from build123d import *

# Parameters (mm, degrees)
SKETCH1_R           = 29.25
SKETCH1_R_2         = 22.025
BOSS_EXTRUDE1_DEPTH = 7
CUT_EXTRUDE1_START  = 7
SKETCH1_3_R         = 1.55
CUT_EXTRUDE1_DEPTH  = 4
SKETCH4_R           = 22.25
SKETCH4_R_2         = 21
BOSS_EXTRUDE2_DEPTH = 1
SKETCH3_R           = 1.55
CUT_EXTRUDE2_DEPTH  = 42.953843686
CHAMFER1_SIZE       = 0.5


with BuildPart() as part:
    # Sketch1 → Boss-Extrude1 (new body)
    with BuildSketch(Plane.XY):
        Circle(SKETCH1_R)
        Circle(SKETCH1_R_2, mode=Mode.SUBTRACT)
    extrude(amount=BOSS_EXTRUDE1_DEPTH)

    # Sketch1<3> → Cut-Extrude1 (cut)
    with BuildSketch(Plane.XY.offset(CUT_EXTRUDE1_START)):
        with Locations((0, 25)):
            Circle(SKETCH1_3_R)
        with Locations((10.847093478, 22.524221698)):
            Circle(SKETCH1_3_R)
        with Locations((19.545787062, 15.587245046)):
            Circle(SKETCH1_3_R)
        with Locations((24.373197805, 5.563023349)):
            Circle(SKETCH1_3_R)
        with Locations((24.373197805, -5.563023349)):
            Circle(SKETCH1_3_R)
        with Locations((19.545787062, -15.587245046)):
            Circle(SKETCH1_3_R)
        with Locations((10.847093478, -22.524221698)):
            Circle(SKETCH1_3_R)
        with Locations((0, -25)):
            Circle(SKETCH1_3_R)
        with Locations((-10.847093478, -22.524221698)):
            Circle(SKETCH1_3_R)
        with Locations((-19.545787062, -15.587245046)):
            Circle(SKETCH1_3_R)
        with Locations((-24.373197805, -5.563023349)):
            Circle(SKETCH1_3_R)
        with Locations((-24.373197805, 5.563023349)):
            Circle(SKETCH1_3_R)
        with Locations((-19.545787062, 15.587245046)):
            Circle(SKETCH1_3_R)
        with Locations((-10.847093478, 22.524221698)):
            Circle(SKETCH1_3_R)
    extrude(amount=-CUT_EXTRUDE1_DEPTH, mode=Mode.SUBTRACT)

    # Sketch4 → Boss-Extrude2 (add)
    with BuildSketch(Plane.XY):
        Circle(SKETCH4_R)
        Circle(SKETCH4_R_2, mode=Mode.SUBTRACT)
    extrude(amount=BOSS_EXTRUDE2_DEPTH)

    # Sketch3 → Cut-Extrude2 (cut, through all)
    with BuildSketch(Plane.XY):
        with Locations((5.89680475, 25.835589673)):
            Circle(SKETCH3_R)
        with Locations((23.875674999, 11.497919087)):
            Circle(SKETCH3_R)
        with Locations((23.875674999, -11.497919087)):
            Circle(SKETCH3_R)
        with Locations((5.89680475, -25.835589673)):
            Circle(SKETCH3_R)
        with Locations((-16.522479749, -20.718534285)):
            Circle(SKETCH3_R)
        with Locations((-26.5, 0)):
            Circle(SKETCH3_R)
        with Locations((-16.522479749, 20.718534285)):
            Circle(SKETCH3_R)
    extrude(amount=CUT_EXTRUDE2_DEPTH, mode=Mode.SUBTRACT)

    # Chamfer1
    chamfer1_edges = [part.edges().sort_by_distance(p)[0] for p in [
        (-22.025, 0, 7),
        (-29.25, 0, 0),
        (-29.25, 0, 7),
    ]]
    chamfer(chamfer1_edges, length=CHAMFER1_SIZE)


solid = part.part
The model under review builds one solid part; all positions refer to its coordinate system, in mm. A direction names the side the tool comes from. Coordinates: 2 decimals unless noted, no trailing zeros. Write each loop counter-clockwise with the first axis right and the second up, starting at its lowest first coordinate (ties: lowest second). Pieces come first, ordered by that corner, then holes. Notation, with made-up numbers: (15.5, 27.25) -> (25.5, 27.25) arc R18 cw to (25.5, 59.25) -> close; hole circle Ø5 at (-6.5, 51.5). An arc over 180 degrees is marked (long way). Answer in a Markdown table with one row per item.
1. We need section C-C, the plane z = 5.25. Give the number of separate pieces and of enclosed holes in the cut face, and give its area (3 significant figures).
Answers below:
| item | result |
|---|---|
| separate pieces | 1 |
| enclosed holes | 22 |
| area | 1,010 mm^2 |
2. We need section B-B, the plane y = 0. State the section outline as (x, z) points (3 decimals).
Answers below:
| item | result |
|---|---|
| outline | (-29.25, 0.5) -> (-28.75, 0) -> (-28.05, 0) -> (-28.05, 7) -> (-28.75, 7) -> (-29.25, 6.5) -> close; (-24.95, 0) -> (-21, 0) -> (-21, 1) -> (-22.025, 1) -> (-22.025, 6.5) -> (-22.525, 7) -> (-24.95, 7) -> close; (21, 0) -> (28.75, 0) -> (29.25, 0.5) -> (29.25, 6.5) -> (28.75, 7) -> (22.525, 7) -> (22.025, 6.5) -> (22.025, 1) -> (21, 1) -> close |
3. For faces 3 (the cylindrical face through (21.008, 6.616, 3.712)), 4 (the cylindrical face through (22.327, 11.566, 3.451)), list the 3-axis set-ups (+Z, -Z, +X, -X, +Y, -Y) from which the entire face can be reached by the end or side of a thin tool; tool diameter is ignored.
Answers below:
| item | result |
|---|---|
| face 3 | +Z |
| face 4 | +Z, -Z |
4. Clearance check with flat-ended pins moving along their axes: pin 1 Ø0.9 at (x, y) = (-19.5, -15) entering from +Z; pin 2 Ø2.5 at (x, y) = (5.9, 25.84) entering from +Z; pin 3 Ø3 at (y, z) = (-9.5, 3) entering from -X. State where each tip first meets the part, or that it passes through.
Answers below:
| item | result |
|---|---|
| pin 1 | stops at z = 3 |
| pin 2 | passes through |
| pin 3 | stops at x = -28.13 |
5. Wall thickness on probe 1 along Y at (x, z) = (24.5, 1); probe 2 along X at (y, z) = (23, 6); probe 3 along X at (y, z) = (-5.5, 3.75): over which ranges is each line inside the solid? List them lowest first. Write a range as [from, to].
Answers below:
| item | result |
|---|---|
| probe 1 | y = [-15.98, -12.92], [-10.08, 10.08], [12.92, 15.98] |
| probe 2 | x = [-18.07, -12.32], [-9.37, 9.37], [12.32, 18.07] |
| probe 3 | x = [-28.73, -25.92], [-22.82, -21.33], [21.33, 22.82], [25.92, 28.73] |
6. We need section A-A, the plane x = 0. State the section outline as (y, z) points (3 decimals), and give its area (4 significant figures).
Answers below:
| item | result |
|---|---|
| outline | (-29.25, 0.5) -> (-28.75, 0) -> (-21, 0) -> (-21, 1) -> (-22.025, 1) -> (-22.025, 6.5) -> (-22.525, 7) -> (-23.45, 7) -> (-23.45, 3) -> (-26.55, 3) -> (-26.55, 7) -> (-28.75, 7) -> (-29.25, 6.5) -> close; (21, 0) -> (28.75, 0) -> (29.25, 0.5) -> (29.25, 6.5) -> (28.75, 7) -> (26.55, 7) -> (26.55, 3) -> (23.45, 3) -> (23.45, 7) -> (22.525, 7) -> (22.025, 6.5) -> (22.025, 1) -> (21, 1) -> close |
| area | 77.65 mm^2 |
7. Draft analysis for pull direction X (two halves, no side actions). For faces 1 (the cylindrical face through (10.645, -20.987, 5.028)), 2 (the flat face through (8.4, -21.2, 7)), state which applies: +X half, -X half, draft (parallel to the pull), parting line (faces both ways), or undercut.
Answers below:
| item | result |
|---|---|
| face 1 | undercut |
| face 2 | draft |
